The figure shows three views and two pictorial views of one solid part (mm, origin at its lowest corner). Answer the questions. A direction names the side the tool comes from. Coordinates: 2 decimals unless noted, no trailing zeros. Order: outer loops, then holes, each group sorted by start corner. A loop starts at its lowest first (then second) coordinate and runs counter-clockwise, first axis right, second up. Notation, with made-up numbers: (-16.5, 76.5) - (-8.5, 76.5) arc R10 cw to (-8.5, 80.5) - close; hole circle Ø7 at (54, -28.5). An arc over 180 degrees is marked (long way). Use one line per item in the form item = value.
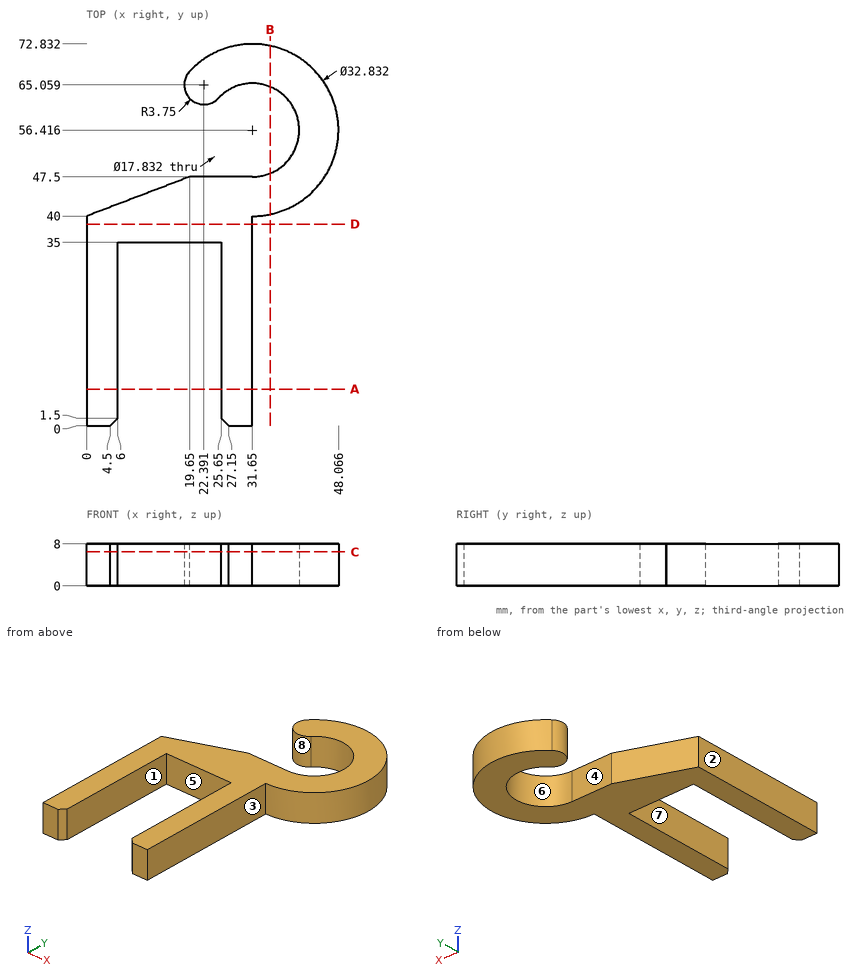
(1) Section D-D, the plane y = 38.5 is taken. Write down the section's boundary in (x, z).
Answer list:
outline = (0, 0) - (31.65, 0) - (31.65, 8) - (0, 8) - close
(2) Given pin 1 Ø3 at (x, z) = (38.5, 3.5) entering from -Y; pin 2 Ø2.5 at (y, z) = (23.5, 5) entering from -X; pin 3 Ø2.5 at (y, z) = (14, 3.5) entering from +X, each flat-ended and moving along its own axis, determine where each tip first touches the part or whether it passes through.
Answer list:
pin_1 = 40.9
pin_2 = 0
pin_3 = 31.65
(3) Section B-B, the plane x = 35 is taken. Write down the section's boundary in (y, z) (1 decimal).
Answer list:
outline = (40.3, 0) - (48.2, 0) - (48.2, 8) - (40.3, 8) - close; (64.7, 0) - (72.5, 0) - (72.5, 8) - (64.7, 8) - close
(4) Which of the six approach directions +Z, -Z, +X, -X, +Y, -Y give full straight-line access (tool end or side, diameter ignored) to the marked faces 1, 2, 3 and 4?
Answer list:
face_1 = +Z, -Z, -Y
face_2 = +Z, -Z, -X, +Y, -Y
face_3 = +Z, -Z, +X, -Y
face_4 = +Z, -Z, -X
(5) The mould has two halves that part along Y. Classify the marked faces 5, 6, 7 and 8: +Y half, -Y half, draft (parallel to the pull), parting line (faces both ways), or undercut.
Answer list:
face_5 = -Y half
face_6 = undercut
face_7 = draft
face_8 = undercut
(6) Straight lines are drawn through the part: L1, parallel to X at y = 16.5, z = 4.75; L2, parallel to Y at x = 38, z = 3.75 (1 decimal); L3, parallel to X at y = 62.5, z = 6. For each, find the intervals that lie inside material, in ascending order.
Answer list:
L1 = 0 to 6, 25.65 to 31.65
L2 = 41.3 to 50.2, 62.7 to 71.6
L3 = 19.65 to 25.13, 38.17 to 46.9
(7) Section A-A, the plane y = 7 is taken. Write down the section's boundary in (x, z), then the cut area to 3 significant figures.
Answer list:
outline = (0, 0) - (6, 0) - (6, 8) - (0, 8) - close; (25.65, 0) - (31.65, 0) - (31.65, 8) - (25.65, 8) - close
area = 96.0 mm2
(8) Section C-C, the plane z = 6.5 is taken. Write down the section's boundary in (x, y).
Answer list:
outline = (0, 0) - (4.5, 0) - (6, 1.5) - (6, 35) - (25.65, 35) - (25.65, 1.5) - (27.15, 0) - (31.65, 0) - (31.65, 40) arc R16.42 ccw (long way) to (19.65, 67.62) arc R3.75 ccw to (25.13, 62.5) arc R8.92 cw (long way) to (31.65, 47.5) - (19.65, 47.5) - (0, 40) - close
